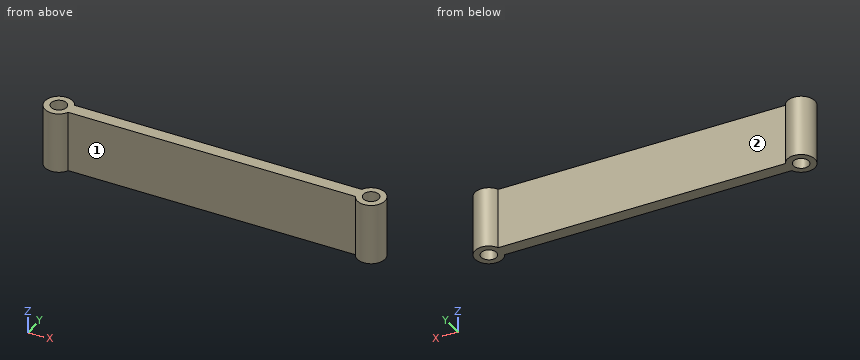
```python
from build123d import *

# Parameters (mm, degrees)
SKETCH1_R           = 3.175
BOSS_EXTRUDE1_DEPTH = 12.7


with BuildPart() as part:
    # Sketch1 → Boss-Extrude1 (new body, symmetric)
    with BuildSketch(Plane.XY):
        with BuildLine():
            Line((5.11953367, 2.54), (121.88046633, 2.54))
            ThreePointArc((121.88046633, 2.54), (132.715, 0), (121.88046633, -2.54))
            Line((121.88046633, -2.54), (5.11953367, -2.54))
            ThreePointArc((5.11953367, -2.54), (-5.715, 0), (5.11953367, 2.54))
        make_face()
        Circle(SKETCH1_R, mode=Mode.SUBTRACT)
        with Locations((127, 0)):
            Circle(SKETCH1_R, mode=Mode.SUBTRACT)
    extrude(amount=BOSS_EXTRUDE1_DEPTH, both=True)


solid = part.part
```
Read the model definition and answer for the solid it produces. Units are mm, in the model's axes. Face numbers are marked on the shaded views. Coordinates: 2 decimals unless noted, no trailing zeros. Loops run counter-clockwise (first coordinate to the right, second up) from the corner with the lowest first, then second, coordinate; pieces in that order, holes last. Notation, with made-up numbers: (-7, 20) -> (20, 20) arc R37 ccw to (20, 58) -> close; hole circle Ø4 at (24.5, 81). An arc over 180 degrees is marked (long way). Return JSON: item names as keys, results as strings.
Item 1: Find section A-A (y = 0). Determine the outline of the cut face in (x, z) (3 decimals).
Answers:
{"outline": "(-5.715, -12.7) -> (-3.175, -12.7) -> (-3.175, 12.7) -> (-5.715, 12.7) -> close; (3.175, -12.7) -> (123.825, -12.7) -> (123.825, 12.7) -> (3.175, 12.7) -> close; (130.175, -12.7) -> (132.715, -12.7) -> (132.715, 12.7) -> (130.175, 12.7) -> close"}
Item 2: Find section D-D (x = 49). Determine the outline of the cut face in (y, z), plus the area to 3 significant figures.
Answers:
{"outline": "(-2.54, -12.7) -> (2.54, -12.7) -> (2.54, 12.7) -> (-2.54, 12.7) -> close", "area": "129 mm2"}
Item 3: Flat-ended cylindrical pins translate along their axes: P1, Ø1.5, axis at y = -3, z = 5.5, coming from the -X side; P2, Ø1, axis at y = -4, z = 6, coming from the -X side; P3, Ø2, axis at x = 117, y = 4.5, coming from the +Z side; P4, Ø12, axis at x = 25.5, z = -1.5, coming from the -Y side. Find the tip coordinate at first contact, or state that the pin passes through.
Answers:
{"P1": "stops at x = -5.25", "P2": "stops at x = -4.52", "P3": "passes through", "P4": "stops at y = -2.54"}
Item 4: For a pull along X with two mould halves and no side action, classify the marked faces 1 and 2 as +X half, -X half, draft (parallel to the pull), parting line (faces both ways), or undercut.
Answers:
{"face 1": "undercut", "face 2": "undercut"}
Item 5: Find the intervals of material crossed by probe 1 along Y at (x, z) = (0, 7.75) (3 decimals); probe 2 along X at (y, z) = (2.75, 10.5); probe 3 along X at (y, z) = (-2, -8), in increasing order.
Answers:
{"probe 1": "y = -5.715 to -3.175, 3.175 to 5.715", "probe 2": "x = -5.01 to -1.59, 1.59 to 5.01, 121.99 to 125.41, 128.59 to 132.01", "probe 3": "x = -5.35 to -2.47, 2.47 to 124.53, 129.47 to 132.35"}
Item 6: Find section C-C (z = -8.75). Determine the outline of the cut face in (x, y) (3 decimals), plus the area to 3 significant figures.
Answers:
{"outline": "(5.12, -2.54) -> (121.88, -2.54) arc R5.715 ccw (long way) to (121.88, 2.54) -> (5.12, 2.54) arc R5.715 ccw (long way) to start; hole circle Ø6.35 at (0, 0); hole circle Ø6.35 at (127, 0)", "area": "731 mm2"}
Item 7: Find section B-B (x = 0). Determine the outline of the cut face in (y, z) (3 decimals), plus the area to 3 significant figures.
Answers:
{"outline": "(-5.715, -12.7) -> (-3.175, -12.7) -> (-3.175, 12.7) -> (-5.715, 12.7) -> close; (3.175, -12.7) -> (5.715, -12.7) -> (5.715, 12.7) -> (3.175, 12.7) -> close", "area": "129 mm2"}
